Autodesk Inventor part; units mm, degrees
ref_plane "YZ Plane" through (0, 0, 0) normal (1, 0, 0) x (0, 1, 0)
ref_plane "XZ Plane" through (0, 0, 0) normal (0, 1, 0) x (-1, 0, 0)
ref_plane "XY Plane" through (0, 0, 0) normal (0, 0, 1) x (1, 0, 0)
sketch "Sketch1" plane through (0, 0, 0) normal (0, 1, 0) x (-1, 0, 0)
  circle A0 centre (0, 19.05) radius 4.1656
  circle A1 centre (0, -19.05) radius 4.1656
  circle A2 centre (-106.68, 0) radius 3.175
  arc A3 (6.35, 19.05) -> (-1.1163, 25.3011) centre (0, 19.05) ccw
  arc A4 (-1.1163, -25.3011) -> (6.35, -19.05) centre (0, -19.05) ccw
  line L0 (0, 19.05) -> (-106.68, 0) construction
  line L1 (-106.68, 0) -> (0, -19.05) construction
  line L2 (-107.7963, -6.2511) -> (-1.1163, -25.3011)
  line L3 (-107.7963, 6.2511) -> (-1.1163, 25.3011)
  line L4 (-132.5233, 0) -> (35.4452, 0) construction
  line L5 (6.35, 19.05) -> (6.35, -19.05)
  arc A5 (-107.7963, 6.2511) -> (-107.7963, -6.2511) centre (-106.68, 0) ccw
  point P0 (0, 0)
  dimension "d0" = 38.1
  dimension "d2" = 19.05
  dimension "d3" = 106.68
  dimension "d4" = 8.3312
  dimension "d5" = 8.3312
  dimension "d6" = 6.35
  dimension "d8" = 12.7
  dimension "d9" = 12.7
  dimension "d10" = 20.249
  dimension "d11" = 6.35
  dimension "d12" = 79.875
  dimension "d13" = 0
  dimension "d14" = 29.0952
  dimension "d15" = 138.8733
extrude "Extrusion1" add sketch "Sketch1" along normal blind 3.175
equation "\"d5\" = d4"
properties part number "x_axis_shaft_support"
Can you work these out from the model? Positions are in its coordinate system, mm. Give positions to 0.01 mm unless a question says otherwise; leave off trailing zeros. Loops run counter-clockwise (first coordinate to the right, second up) from the corner with the lowest first, then second, coordinate; pieces in that order, holes last. Notation, with made-up numbers: M 42,18.25 L 60,18.25 A23 cw 60,40.25 Z; hole C 25.25,84.25 d9. An arc over 180 degrees is marked long. Use CSV: the item, a comma, the result in double quotes. Start each with the question number.
1. Imagine slicing it at C-C, the plane x = 106.68. Write out the boundary of the cut face in (y, z) (3 decimals), plus the area to 3 significant figures.
2. Imagine slicing it at B-B, the plane x = 0. Write out the boundary of the cut face in (y, z) (3 decimals).
3. If I drill on L1, parallel to Z at x = 0, y = 2.5; L2, parallel to Z at x = 2, y = 0.85; L3, parallel to Z at x = 106, y = 0.75, over which ranges is the centre line in solid material (lowest first)?
4. Imagine slicing it at A-A, the plane y = 2.4. Write out the boundary of the cut face in (x, z) (3 decimals).
5. If we mould it in two halves opening along X, with no side actions, what happens to faces 1 (the face through (-6.35, 2, 0)), 2 (the face through (103.65, 1.57, -0.95)), 3 (the face through (55.203, 1.565, -15.643))? For each: released by +X, released by -X, zero draft, split by the parting line, or undercut.
6. Imagine slicing it at D-D, the plane z = 5. Write out the boundary of the cut face in (x, y) (3 decimals).
7. For P1, Ø6.5, axis at x = 0, z = -19.05, coming from the +Y side, with a flat end and sliding along its axis, tell me the tip position at first contact or that it passes through.
Response values:
1,outline,"M 0,-6.45 L 3.175,-6.45 L 3.175,-3.175 L 0,-3.175 Z; M 0,3.175 L 3.175,3.175 L 3.175,6.45 L 0,6.45 Z"
1,area,"20.8 mm^2"
2,outline,"M 0,-25.4 L 3.175,-25.4 L 3.175,-23.216 L 0,-23.216 Z; M 0,-14.884 L 3.175,-14.884 L 3.175,14.884 L 0,14.884 Z; M 0,23.216 L 3.175,23.216 L 3.175,25.4 L 0,25.4 Z"
3,L1,"-25.4 to -23.22, -14.88 to 14.88, 23.22 to 25.4"
3,L2,"-25.14 to -22.7, -15.4 to 15.4, 22.7 to 25.14"
3,L3,"-6.57 to -3.1, 3.1 to 6.57"
4,outline,"M -6.35,-19.05 A6.35 ccw 1.116,-25.301 L 107.796,-6.251 A6.35 ccw 107.796,6.251 L 1.116,25.301 A6.35 ccw -6.35,19.05 Z; hole C 0,-19.05 d8.331; hole C 0,19.05 d8.331; hole C 106.68,0 d6.35"
5,face 1,"released by -X"
5,face 2,"undercut"
5,face 3,"released by +X"
6,outline,"M -6.35,0 L 110.594,0 L 110.594,3.175 L -6.35,3.175 Z"
7,P1,"through"
